from build123d import *

# Parameters (mm, degrees)
SKETCH_1_W          = 160
SKETCH_1_H          = 160
EXTRUDE_1_DEPTH     = 14
SKETCH_2_R          = 15
SKETCH_2_R_2        = 1.4
CUT_EXTRUDE_1_DEPTH = 16
SKETCH_3_R          = 2.6
CUT_EXTRUDE_2_DEPTH = 20
FILLET_1_R          = 10
SKETCH_5_R          = 3.5
CUT_EXTRUDE_3_DEPTH = 4
CUT_EXTRUDE_4_DEPTH = 20
SKETCH_7_R          = 2.5
CUT_EXTRUDE_5_DEPTH = 20
FILLET_2_R          = 5
FILLET_3_R          = 5


with BuildPart() as part:
    # 草图1 → 凸台-拉伸1 (new body)
    with BuildSketch(Plane(origin=(0, 0, 0), x_dir=(1, 0, 0), z_dir=(0, 1, 0))):
        with Locations((80, 80)):
            Rectangle(SKETCH_1_W, SKETCH_1_H)
    extrude(amount=EXTRUDE_1_DEPTH)

    # 草图2 → 切除-拉伸1 (cut)
    with BuildSketch(Plane(origin=(0, 14, 0), x_dir=(1, 0, 0), z_dir=(0, 1, 0))):
        with Locations(Location((80, 80, 0), (0, 0, 270))):
            Circle(SKETCH_2_R)
        with Locations(Location((60, 80, 0), (0, 0, 270))):
            Circle(SKETCH_2_R_2)
        with Locations(Location((70, 97.320508076, 0), (0, 0, 270))):
            Circle(SKETCH_2_R_2)
        with Locations(Location((90, 97.320508076, 0), (0, 0, 270))):
            Circle(SKETCH_2_R_2)
        with Locations(Location((100, 80, 0), (0, 0, 270))):
            Circle(SKETCH_2_R_2)
        with Locations(Location((90, 62.679491924, 0), (0, 0, 270))):
            Circle(SKETCH_2_R_2)
        with Locations(Location((70, 62.679491924, 0), (0, 0, 270))):
            Circle(SKETCH_2_R_2)
    extrude(amount=-CUT_EXTRUDE_1_DEPTH, mode=Mode.SUBTRACT)

    # 草图3 → 切除-拉伸2 (cut)
    with BuildSketch(Plane(origin=(0, 14, 0), x_dir=(1, 0, 0), z_dir=(0, 1, 0))):
        with Locations(Location((10, 150, 0), (0, 0, 270))):
            Circle(SKETCH_3_R)
        with Locations(Location((150, 150, 0), (0, 0, 90))):
            Circle(SKETCH_3_R)
        with Locations(Location((150, 10, 0), (0, 0, 270))):
            Circle(SKETCH_3_R)
        with Locations(Location((10, 10, 0), (0, 0, 90))):
            Circle(SKETCH_3_R)
    extrude(amount=-CUT_EXTRUDE_2_DEPTH, mode=Mode.SUBTRACT)

    # 圆角1
    fillet_1_edges = [part.edges().sort_by_distance(p)[0] for p in [
        (0, 7, -160),
        (160, 7, -160),
        (160, 7, 0),
        (0, 7, 0),
    ]]
    fillet(fillet_1_edges, radius=FILLET_1_R)

    # 草图5 → 切除-拉伸3 (cut)
    with BuildSketch(Plane.XZ):
        with Locations(Location((100, -80, 0), (0, 0, 270))):
            Circle(SKETCH_5_R)
        with Locations(Location((90, -97.320508076, 0), (0, 0, 270))):
            Circle(SKETCH_5_R)
        with Locations(Location((70, -97.320508076, 0), (0, 0, 270))):
            Circle(SKETCH_5_R)
        with Locations(Location((60, -80, 0), (0, 0, 270))):
            Circle(SKETCH_5_R)
        with Locations(Location((70, -62.679491924, 0), (0, 0, 270))):
            Circle(SKETCH_5_R)
        with Locations(Location((90, -62.679491924, 0), (0, 0, 270))):
            Circle(SKETCH_5_R)
    extrude(amount=-CUT_EXTRUDE_3_DEPTH, mode=Mode.SUBTRACT)

    # 草图6 → 切除-拉伸4 (cut)
    with BuildSketch(Plane(origin=(0, 14, 0), x_dir=(1, 0, 0), z_dir=(0, 1, 0))):
        with BuildLine():
            ThreePointArc((67.5, 143.786754111), (34.038059223, 125.961940777), (16.213245889, 92.5))
            Line((16.213245889, 92.5), (42.003289616, 92.5))
            ThreePointArc((42.003289616, 92.5), (51.715728753, 108.284271247), (67.5, 117.996710384))
            Line((67.5, 117.996710384), (67.5, 143.786754111))
        make_face()
        with BuildLine():
            ThreePointArc((143.786754111, 92.5), (125.961940777, 125.961940777), (92.5, 143.786754111))
            Line((92.5, 143.786754111), (92.5, 117.996710384))
            ThreePointArc((92.5, 117.996710384), (108.284271247, 108.284271247), (117.996710384, 92.5))
            Line((117.996710384, 92.5), (143.786754111, 92.5))
        make_face()
        with BuildLine():
            Line((92.5, 42.003289616), (92.5, 16.213245889))
            ThreePointArc((92.5, 16.213245889), (125.961940777, 34.038059223), (143.786754111, 67.5))
            Line((143.786754111, 67.5), (117.996710384, 67.5))
            ThreePointArc((117.996710384, 67.5), (108.284271247, 51.715728753), (92.5, 42.003289616))
        make_face()
        with BuildLine():
            Line((42.003289616, 67.5), (16.213245889, 67.5))
            ThreePointArc((16.213245889, 67.5), (34.038059223, 34.038059223), (67.5, 16.213245889))
            Line((67.5, 16.213245889), (67.5, 42.003289616))
            ThreePointArc((67.5, 42.003289616), (51.715728753, 51.715728753), (42.003289616, 67.5))
        make_face()
    extrude(amount=-CUT_EXTRUDE_4_DEPTH, mode=Mode.SUBTRACT)

    # 草图7 → 切除-拉伸5 (cut)
    with BuildSketch(Plane(origin=(0, 14, 0), x_dir=(1, 0, 0), z_dir=(0, 1, 0))):
        with Locations(Location((110.973206237, 60.993261842, 0), (0, 0, 270))):
            Circle(SKETCH_7_R)
    extrude(amount=-CUT_EXTRUDE_5_DEPTH, mode=Mode.SUBTRACT)

    # 圆角2
    fillet_2_edges = [part.edges().sort_by_distance(p)[0] for p in [
        (67.5, 7, -143.786754111),
        (67.5, 7, -117.996710384),
        (42.003289616, 7, -92.5),
        (16.213245889, 7, -92.5),
    ]]
    fillet(fillet_2_edges, radius=FILLET_2_R)

    # 圆角3
    fillet_3_edges = [part.edges().sort_by_distance(p)[0] for p in [
        (16.213245889, 7, -67.5),
        (42.003289616, 7, -67.5),
        (67.5, 7, -42.003289616),
        (67.5, 7, -16.213245889),
        (92.5, 7, -16.213245889),
        (92.5, 7, -42.003289616),
        (117.996710384, 7, -67.5),
        (143.786754111, 7, -67.5),
        (143.786754111, 7, -92.5),
        (117.996710384, 7, -92.5),
        (92.5, 7, -117.996710384),
        (92.5, 7, -143.786754111),
    ]]
    fillet(fillet_3_edges, radius=FILLET_3_R)


solid = part.part
Part model, mm, in its own coordinate system. A direction names the side the tool comes from. Coordinates: 2 decimals unless noted, no trailing zeros. Order: outer loops, then holes, each group sorted by start corner. A loop starts at its lowest first (then second) coordinate and runs counter-clockwise, first axis right, second up. Notation, with made-up numbers: M 1.5,0.25 L 24.5,0.25 A21 cw 24.5,18.25 Z; hole C -20.5,4.5 d4. An arc over 180 degrees is marked long. Use a Markdown table: item, result.
(1) Cut at C-C on y = 11. State how many separate pieces and enclosed holes the cut face has, then the cut area to 3 significant figures.
A:
| item | result |
|---|---|
| separate pieces | 1 |
| enclosed holes | 16 |
| area | 19,000 mm^2 |
(2) Flat gauge pins, fed straight in: pin 1 (6.5 mm diameter, centred on x = 90, z = -97.32, fed in from -Y); pin 2 (3.5 mm diameter, centred on x = 100, z = -80, fed in from +Y). Where does each tip first touch, or does it go through?
A:
| item | result |
|---|---|
| pin 1 | stops at y = 4 |
| pin 2 | stops at y = 14 |
(3) Tool access for faces 1 (the cylindrical face through (96.895, 1.972, -81.615)), 2 (the cylindrical face through (66.69, 6.9, -118.73)), 3 (the flat face through (61.1, 14, -81.1)): list every direction of +Z, -Z, +X, -X, +Y, -Y with a clear straight run to the whole face (end or side of a thin tool).
A:
| item | result |
|---|---|
| face 1 | -Y |
| face 2 | +Y, -Y |
| face 3 | +Z, -Z, +X, -X, +Y |
(4) Probe L1, parallel to X at y = 5, z = -150; L2, parallel to X at y = 10.25, z = -34; L3, parallel to Z at x = 52.5, y = 1.75. List the from-to ranges inside material, lowest first.
A:
| item | result |
|---|---|
| L1 | x = 0 to 7.4, 12.6 to 147.4, 152.6 to 160 |
| L2 | x = 0 to 34.08, 67.5 to 92.5, 125.92 to 160 |
| L3 | z = -160 to -138.9, -109.05 to -50.95, -21.1 to 0 |
(5) Pull direction Z, two halves, no side cores. Call faces 4 (the cylindrical face through (151, 7.1, -152.4)), 5 (the flat face through (160, 7, -79)), 6 (the cylindrical face through (2.85, 7.1, -156.99)): released by +Z, released by -Z, zero draft, split by the parting line, or undercut.
A:
| item | result |
|---|---|
| face 4 | undercut |
| face 5 | zero draft |
| face 6 | released by -Z |
(6) Cut at B-B on z = -86.5. Write the cut outline in (x, y).
A:
| item | result |
|---|---|
| outline | M 0,0 L 66.48,0 L 66.48,14 L 0,14 Z; M 93.52,0 L 160,0 L 160,14 L 93.52,14 Z |
(7) Cut at A-A on x = 80. Write the cut outline in (y, z), then the cut area to 3 significant figures.
A:
| item | result |
|---|---|
| outline | M 0,-160 L 14,-160 L 14,-95 L 0,-95 Z; M 0,-65 L 14,-65 L 14,0 L 0,0 Z |
| area | 1,820 mm^2 |
